from build123d import *

# Parameters (mm, degrees)
BOSS_EXTRUDE1_DEPTH     = 3
SKETCH2_R               = 2.5
CUT_EXTRUDE1_DEPTH      = 4
LPATTERN1_COUNT         = 2
LPATTERN1_PITCH         = 40
LPATTERN1_COUNT_DIR2    = 2
LPATTERN1_PITCH_DIR2    = 20
MIRROR1_COPY_1_SKETCH_R = 2.5
MIRROR1_COPY_1_DEPTH    = 4
MIRROR1_COPY_2_SKETCH_R = 2.5
MIRROR1_COPY_2_DEPTH    = 4
MIRROR1_COPY_3_SKETCH_R = 2.5
MIRROR1_COPY_3_DEPTH    = 4
SKETCH3_R               = 2.5
CUT_EXTRUDE2_DEPTH      = 4
FILLET1_R               = 5


with BuildPart() as part:
    # Sketch1 → Boss-Extrude1 (new body)
    with BuildSketch(Plane.XY):
        Polygon((-110, 20), (-110, -20), (-45, -50), (45, -50), (110, -20), (110, 20), (45, 50), (-45, 50), align=None)
    extrude(amount=BOSS_EXTRUDE1_DEPTH)

    # Sketch2 → Cut-Extrude1 (cut, through all)
    with BuildSketch(Plane.XY.offset(3)):
        with Locations((60, 10)):
            Circle(SKETCH2_R)
    cut_extrude1 = extrude(amount=-CUT_EXTRUDE1_DEPTH, mode=Mode.SUBTRACT)

    # LPattern1: Cut-Extrude1 2 × 2
    with Locations(*[(i * LPATTERN1_PITCH, -j * LPATTERN1_PITCH_DIR2, 0) for i in range(LPATTERN1_COUNT) for j in range(LPATTERN1_COUNT_DIR2) if (i, j) != (0, 0)]):
        add(cut_extrude1, mode=Mode.SUBTRACT)

    # Mirror1: Cut-Extrude1 across plane
    add(cut_extrude1.mirror(Plane(origin=(0, 0, 0), x_dir=(0, 0, 1), z_dir=(1, 0, 0))), mode=Mode.SUBTRACT)

    # Mirror1 copy 1 sketch → Mirror1 copy 1 (cut, through all)
    with BuildSketch(Plane(origin=(0, -20, 3), x_dir=(-1, 0, 0), z_dir=(0, 0, 1))):
        with Locations((60, -10)):
            Circle(MIRROR1_COPY_1_SKETCH_R)
    extrude(amount=-MIRROR1_COPY_1_DEPTH, mode=Mode.SUBTRACT)

    # Mirror1 copy 2 sketch → Mirror1 copy 2 (cut, through all)
    with BuildSketch(Plane(origin=(-40, 0, 3), x_dir=(-1, 0, 0), z_dir=(0, 0, 1))):
        with Locations((60, -10)):
            Circle(MIRROR1_COPY_2_SKETCH_R)
    extrude(amount=-MIRROR1_COPY_2_DEPTH, mode=Mode.SUBTRACT)

    # Mirror1 copy 3 sketch → Mirror1 copy 3 (cut, through all)
    with BuildSketch(Plane(origin=(-40, -20, 3), x_dir=(-1, 0, 0), z_dir=(0, 0, 1))):
        with Locations((60, -10)):
            Circle(MIRROR1_COPY_3_SKETCH_R)
    extrude(amount=-MIRROR1_COPY_3_DEPTH, mode=Mode.SUBTRACT)

    # Sketch3 → Cut-Extrude2 (cut, through all)
    with BuildSketch(Plane.XY.offset(3)):
        with Locations((20, 40)):
            Circle(SKETCH3_R)
        with Locations((-20, 40)):
            Circle(SKETCH3_R)
    cut_extrude2 = extrude(amount=-CUT_EXTRUDE2_DEPTH, mode=Mode.SUBTRACT)

    # Mirror2: Cut-Extrude2 across plane
    add(cut_extrude2.mirror(Plane.ZX), mode=Mode.SUBTRACT)

    # Fillet1
    fillet1_edges = [part.edges().sort_by_distance(p)[0] for p in [
        (-45, 50, 1.5),
        (45, 50, 1.5),
        (110, 20, 1.5),
        (110, -20, 1.5),
        (45, -50, 1.5),
        (-45, -50, 1.5),
        (-110, -20, 1.5),
        (-110, 20, 1.5),
    ]]
    fillet(fillet1_edges, radius=FILLET1_R)


solid = part.part
Work out the finished part from the listing and answer in its coordinate system (mm). Give positions to 0.01 mm unless a question says otherwise; leave off trailing zeros. Order: outer loops, then holes, each group sorted by start corner. A loop starts at its lowest first (then second) coordinate and runs counter-clockwise, first axis right, second up. Notation, with made-up numbers: (89, 15.5) - (128, 15.5) arc R14 cw to (128, 29.5) - close; hole circle Ø5 at (53.25, -8.5). An arc over 180 degrees is marked (long way). Answer as CSV lines item,"result". Start each with the question number.
Q1. The mould has two halves that part along X. Classify faces 1 (the face through (-76.119, 35.638, 1.479)), 2 (the face through (-101.15, 12.22, 1.52)), 3 (the face through (76.974, 35.243, 1.479)): +X half, -X half, draft (parallel to the pull), parting line (faces both ways), or undercut.
Q2. Given pin 1 Ø6.5 at (x, y) = (-60, -10) entering from +Z; pin 2 Ø4 at (x, y) = (60, -10) entering from +Z, each flat-ended and moving along its own axis, determine where each tip first touches the part or whether it passes through.
Q3. Find the intervals of material crossed by L1, parallel to X at y = -12, z = 1.4; L2, parallel to Y at x = 60, z = 2.1; L3, parallel to Y at x = -98.5, z = 0.7, in increasing order. Write a range as [from, to].
Q4. The part is cut by section B-B (x = 20). Write down the section's boundary in (y, z), then the cut area to 3 significant figures.
Q5. The part is cut by section A-A (z = 2). Give the number of separate pieces and of enclosed holes in the cut face, then the cut area to 3 significant figures.
Q6. The part is cut by section C-C (y = 40). Write down the section's boundary in (x, z), then the cut area to 3 significant figures.
Q7. The part is cut by section D-D (y = 24). Write down the section's boundary in (x, z).
Check result:
1,face 1,"-X half"
1,face 2,"undercut"
1,face 3,"+X half"
2,pin 1,"stops at z = 3"
2,pin 2,"passes through"
3,L1,"x = [-110, -101.5], [-98.5, -61.5], [-58.5, 58.5], [61.5, 98.5], [101.5, 110]"
3,L2,"y = [-43.08, -12.5], [-7.5, 7.5], [12.5, 43.08]"
3,L3,"y = [-25.31, -12], [-8, 8], [12, 25.31]"
4,outline,"(-50, 0) - (-42.5, 0) - (-42.5, 3) - (-50, 3) - close; (-37.5, 0) - (37.5, 0) - (37.5, 3) - (-37.5, 3) - close; (42.5, 0) - (50, 0) - (50, 3) - (42.5, 3) - close"
4,area,"270 mm²"
5,separate pieces,"1"
5,enclosed holes,"12"
5,area,"17,900 mm²"
6,outline,"(-66.67, 0) - (-22.5, 0) - (-22.5, 3) - (-66.67, 3) - close; (-17.5, 0) - (17.5, 0) - (17.5, 3) - (-17.5, 3) - close; (22.5, 0) - (66.67, 0) - (66.67, 3) - (22.5, 3) - close"
6,area,"370 mm²"
7,outline,"(-101.33, 0) - (101.33, 0) - (101.33, 3) - (-101.33, 3) - close"
